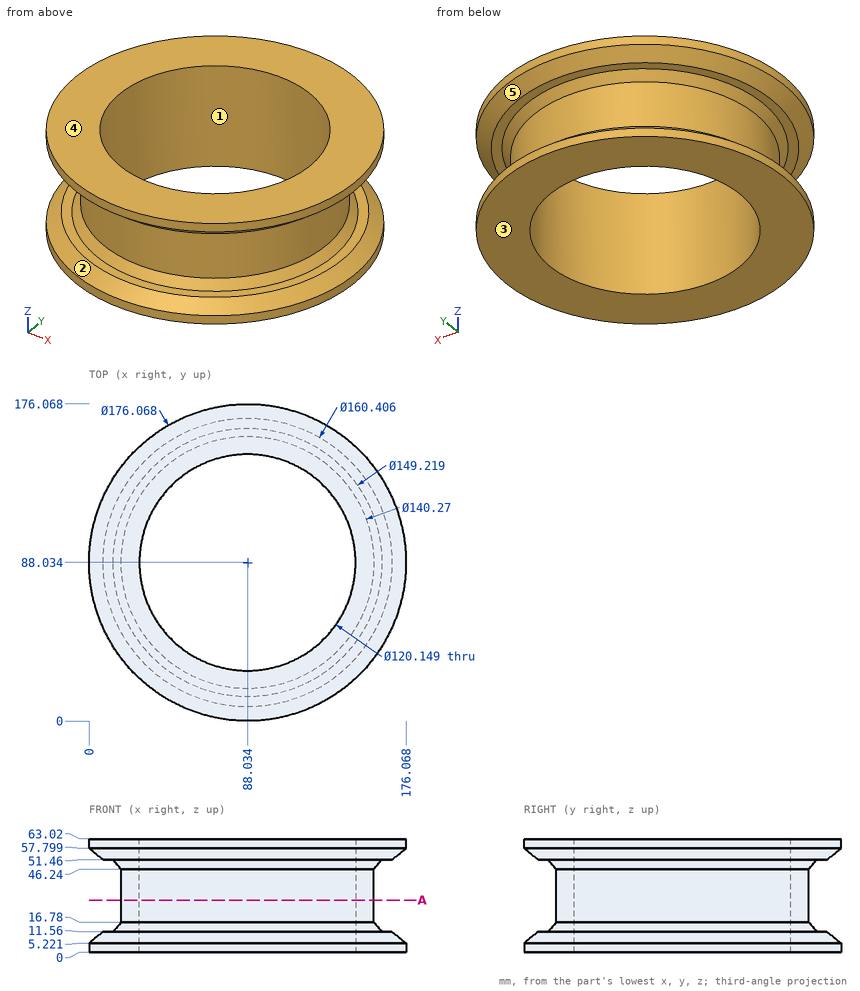
Answer from the drawing. Dimensions are ordinates in mm from the lowest x, y and z of the part. A direction names the side the tool comes from. Coordinates: 2 decimals unless noted, no trailing zeros. Loops run counter-clockwise (first coordinate to the right, second up) from the corner with the lowest first, then second, coordinate; pieces in that order, holes last. Notation, with made-up numbers: (-16.75, -30.5) -> (-10.75, -30.5) arc R27 ccw to (-10.75, -7.5) -> close; hole circle Ø11 at (59, 5.5). An arc over 180 degrees is marked (long way). Return JSON: item names as keys, results as strings.
Item 1: Find section A-A (z = 29). Determine the outline of the cut face in (x, y) (1 decimal).
Answers:
{"outline": "circle Ø140.3 at (88, 88); hole circle Ø120.1 at (88, 88)"}
Item 2: Flat-ended cylindrical pins translate along their axes: P1, Ø4, axis at y = 44, z = 31, coming from the -X side; P2, Ø10, axis at x = 39, z = 7, coming from the -Y side (1 decimal); P3, Ø8, axis at y = 37, z = 54, coming from the -X side. Find the tip coordinate at first contact, or state that the pin passes through.
Answers:
{"P1": "stops at x = 31.89", "P2": "stops at y = 12", "P3": "stops at x = 15.39"}
Item 3: For a pull along Y with two mould halves and no side action, classify the marked faces 1, 2 and 3 as +Y half, -Y half, draft (parallel to the pull), parting line (faces both ways), or undercut.
Answers:
{"face 1": "undercut", "face 2": "parting line", "face 3": "draft"}
Item 4: Find the intervals of material crossed by probe 1 along Z at (x, y) = (150, 136.5); probe 2 along Y at (x, z) = (62.5, 54) (1 decimal); probe 3 along Y at (x, z) = (39, 20.5) (1 decimal), in increasing order.
Answers:
{"probe 1": "z = 0 to 11.56, 51.46 to 63.02", "probe 2": "y = 8.7 to 33.7, 142.4 to 167.4", "probe 3": "y = 37.9 to 53.3, 122.7 to 138.2"}
Item 5: For the marked faces 4 and 5, determine the directions among +Z, -Z, +X, -X, +Y, -Y from which every point of the face is accessible in a straight line to the end or side of a thin tool.
Answers:
{"face 4": "+Z, +X, -X, +Y, -Y", "face 5": "none"}
